```python
from build123d import *

# Parameters (mm, degrees)
SKETCH4_W                        = 25.4
SKETCH4_H                        = 25.4
SKETCH4_W_2                      = 15.875
SKETCH4_H_2                      = 15.875
BOSS_EXTRUDE1_DEPTH              = 196.85
F_0_257_DIAMETER_HOLE1_D         = 6.5278
F_0_257_DIAMETER_HOLE2_D         = 6.5278
F_0_257_DIAMETER_HOLE3_D         = 6.5278
F_17_64_0_26563_DIAMETER_HOLE1_D = 6.747002


with BuildPart() as part:
    # Sketch4 → Boss-Extrude1 (new body, symmetric)
    with BuildSketch(Plane.XY):
        Rectangle(SKETCH4_W, SKETCH4_H)
        Rectangle(SKETCH4_W_2, SKETCH4_H_2, mode=Mode.SUBTRACT)
    extrude(amount=BOSS_EXTRUDE1_DEPTH, both=True)

    # F (0.257) Diameter Hole1 (through all)
    with Locations(Plane.ZY.offset(12.7)):
        with Locations((-104.775, 0), (-123.825, 0), (-168.275, 0), (-187.325, 0)):
            Hole(F_0_257_DIAMETER_HOLE1_D / 2)

    # F (0.257) Diameter Hole2 (through all)
    with Locations(Plane(origin=(0, 12.7, 0), x_dir=(1, 0, 0), z_dir=(0, 1, 0))):
        with Locations((0, -177.8), (0, -158.75)):
            Hole(F_0_257_DIAMETER_HOLE2_D / 2)

    # F (0.257) Diameter Hole3 (through all)
    with Locations(Plane.ZY.offset(12.7)):
        with Locations((168.275, 0), (-44.45, 0)):
            Hole(F_0_257_DIAMETER_HOLE3_D / 2)

    # 17/64 (0.26563) Diameter Hole1 (through all)
    with Locations(Plane.ZY.offset(12.7)):
        with Locations((-146.05, 0)):
            Hole(F_17_64_0_26563_DIAMETER_HOLE1_D / 2)


solid = part.part
```
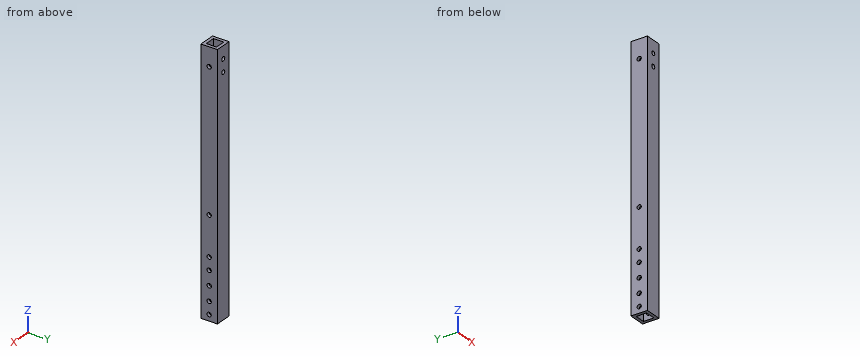
Part model, mm, in its own coordinate system. Round coordinates to 2 decimals unless told otherwise and drop trailing zeros. Loops run counter-clockwise (first coordinate to the right, second up) from the corner with the lowest first, then second, coordinate; pieces in that order, holes last. Notation, with made-up numbers: (21.25, 5) -> (65.25, 5) arc R27 cw to (65.25, 33) -> close; hole circle Ø5 at (-25.75, 9). An arc over 180 degrees is marked (long way). Use one line per item in the form item = value. Start each with the question number.
Item 1: Drill centre lines: line 1 along Z through (x, y) = (0, 8.25); line 2 along Z through (x, y) = (-0.5, 11); line 3 along Y through (x, z) = (-7, 138.5). Where is each one in solid material? Low to high.
Item 2: Band-saw the part on C-C (y = 0). Give the number of separate pieces and of enclosed holes in the cut face, plus the area to 3 significant figures.
Item 3: Band-saw the part on D-D (z = -146.05). List the corners of the cut face in (x, y), plus the area to 3 significant figures.
Item 4: Band-saw the part on B-B (z = 92.5). List the corners of the cut face in (x, y).
Item 5: Band-saw the part on A-A (z = -44.45). List the corners of the cut face in (x, y).
Item 6: Drop a flat-ended pin along its axis: pin 1 Ø4 at (y, z) = (0, -168.275) entering from -X. Give the stop position or say it passes through.
Data:
q1.line_1 = -196.85 to 155.49, 162.01 to 174.54, 181.06 to 196.85
q1.line_2 = -196.85 to 155.52, 161.98 to 174.57, 181.03 to 196.85
q1.line_3 = -12.7 to -7.94, 7.94 to 12.7
q2.separate_pieces = 16
q2.enclosed_holes = 0
q2.area = 3,310 mm^2
q3.outline = (-12.7, -12.7) -> (12.7, -12.7) -> (12.7, -3.37) -> (7.94, -3.37) -> (7.94, -7.94) -> (-7.94, -7.94) -> (-7.94, -3.37) -> (-12.7, -3.37) -> close; (-12.7, 3.37) -> (-7.94, 3.37) -> (-7.94, 7.94) -> (7.94, 7.94) -> (7.94, 3.37) -> (12.7, 3.37) -> (12.7, 12.7) -> (-12.7, 12.7) -> close
q3.area = 329 mm^2
q4.outline = (-12.7, -12.7) -> (12.7, -12.7) -> (12.7, 12.7) -> (-12.7, 12.7) -> close; hole (-7.94, -7.94) -> (7.94, -7.94) -> (7.94, 7.94) -> (-7.94, 7.94) -> close
q5.outline = (-12.7, -12.7) -> (12.7, -12.7) -> (12.7, -3.26) -> (7.94, -3.26) -> (7.94, -7.94) -> (-7.94, -7.94) -> (-7.94, -3.26) -> (-12.7, -3.26) -> close; (-12.7, 3.26) -> (-7.94, 3.26) -> (-7.94, 7.94) -> (7.94, 7.94) -> (7.94, 3.26) -> (12.7, 3.26) -> (12.7, 12.7) -> (-12.7, 12.7) -> close
q6.pin_1 = through
